Input: part model. Units: mm. Frame: model coordinates. Coordinates: 2 decimals unless noted, no trailing zeros. Write each loop counter-clockwise with the first axis right and the second up, starting at its lowest first coordinate (ties: lowest second). Pieces come first, ordered by that corner, then holes. Notation, with made-up numbers: (68, 12) - (115, 12) arc R24 ccw to (115, 35) - close; hole circle Ø10 at (38, -28). An arc over 180 degrees is marked (long way). Use CSV: the item, a comma, the result in double quotes.
Autodesk Inventor part; units mm, degrees
ref_plane "YZ Plane" through (0, 0, 0) normal (1, 0, 0) x (0, 1, 0)
ref_plane "XZ Plane" through (0, 0, 0) normal (0, 1, 0) x (-1, 0, 0)
ref_plane "XY Plane" through (0, 0, 0) normal (0, 0, 1) x (1, 0, 0)
sketch "Sketch1" plane through (0, 0, 0) normal (0, 1, 0) x (-1, 0, 0)
  line L0 (0, 0) -> (152.4, 0)
  line L1 (152.4, 0) -> (152.4, 203.2)
  line L2 (152.4, 203.2) -> (0, 203.2)
  line L3 (0, 203.2) -> (0, 0)
  circle A0 centre (12.7, 190.5) radius 7.9375
  circle A1 centre (139.7, 190.5) radius 7.9375
  circle A2 centre (139.7, 12.7) radius 7.9375
  circle A3 centre (12.7, 12.7) radius 7.9375
  circle A4 centre (114.3, 190.5) radius 3.302
  circle A5 centre (38.1, 190.5) radius 3.302
  circle A6 centre (114.3, 12.7) radius 3.302
  circle A7 centre (38.1, 12.7) radius 3.302
  circle A8 centre (139.7, 139.7) radius 3.302
  circle A9 centre (139.7, 63.5) radius 3.302
  circle A10 centre (20.32, 168.148) radius 1.524
  circle A11 centre (20.32, 153.924) radius 1.524
  circle A12 centre (20.32, 128.524) radius 1.524
  circle A13 centre (20.32, 114.3) radius 1.524
  circle A14 centre (20.32, 88.9) radius 1.524
  circle A15 centre (20.32, 74.676) radius 1.524
  circle A16 centre (20.32, 49.276) radius 1.524
  circle A17 centre (20.32, 35.052) radius 1.524
  line L4 (152.4, 203.2) -> (139.7, 203.2)
  line L5 (139.7, 203.2) -> (139.7, 200.025)
  line L6 (139.7, 200.025) -> (152.4, 200.025)
  line L7 (152.4, 200.025) -> (152.4, 203.2)
  line L8 (127, 203.2) -> (114.3, 203.2)
  line L9 (114.3, 203.2) -> (114.3, 200.025)
  line L10 (114.3, 200.025) -> (127, 200.025)
  line L11 (127, 200.025) -> (127, 203.2)
  line L12 (101.6, 203.2) -> (88.9, 203.2)
  line L13 (88.9, 203.2) -> (88.9, 200.025)
  line L14 (88.9, 200.025) -> (101.6, 200.025)
  line L15 (101.6, 200.025) -> (101.6, 203.2)
  line L16 (76.2, 203.2) -> (63.5, 203.2)
  line L17 (63.5, 203.2) -> (63.5, 200.025)
  line L18 (63.5, 200.025) -> (76.2, 200.025)
  line L19 (76.2, 200.025) -> (76.2, 203.2)
  line L20 (50.8, 203.2) -> (38.1, 203.2)
  line L21 (38.1, 203.2) -> (38.1, 200.025)
  line L22 (38.1, 200.025) -> (50.8, 200.025)
  line L23 (50.8, 200.025) -> (50.8, 203.2)
  line L24 (25.4, 203.2) -> (12.7, 203.2)
  line L25 (12.7, 203.2) -> (12.7, 200.025)
  line L26 (12.7, 200.025) -> (25.4, 200.025)
  line L27 (25.4, 200.025) -> (25.4, 203.2)
  line L28 (152.4, 0) -> (139.7, 0)
  line L29 (139.7, 0) -> (139.7, 3.175)
  line L30 (139.7, 3.175) -> (152.4, 3.175)
  line L31 (152.4, 3.175) -> (152.4, 0)
  line L32 (127, 0) -> (114.3, 0)
  line L33 (114.3, 0) -> (114.3, 3.175)
  line L34 (114.3, 3.175) -> (127, 3.175)
  line L35 (127, 3.175) -> (127, 0)
  line L36 (101.6, 0) -> (88.9, 0)
  line L37 (88.9, 0) -> (88.9, 3.175)
  line L38 (88.9, 3.175) -> (101.6, 3.175)
  line L39 (101.6, 3.175) -> (101.6, 0)
  line L40 (76.2, 0) -> (63.5, 0)
  line L41 (63.5, 0) -> (63.5, 3.175)
  line L42 (63.5, 3.175) -> (76.2, 3.175)
  line L43 (76.2, 3.175) -> (76.2, 0)
  line L44 (50.8, 0) -> (38.1, 0)
  line L45 (38.1, 0) -> (38.1, 3.175)
  line L46 (38.1, 3.175) -> (50.8, 3.175)
  line L47 (50.8, 3.175) -> (50.8, 0)
  line L48 (25.4, 0) -> (12.7, 0)
  line L49 (12.7, 0) -> (12.7, 3.175)
  line L50 (12.7, 3.175) -> (25.4, 3.175)
  line L51 (25.4, 3.175) -> (25.4, 0)
  line L52 (152.4, 187.325) -> (149.225, 187.325)
  line L53 (149.225, 187.325) -> (149.225, 174.625)
  line L54 (149.225, 174.625) -> (152.4, 174.625)
  line L55 (152.4, 174.625) -> (152.4, 187.325)
  line L56 (152.4, 161.925) -> (149.225, 161.925)
  line L57 (149.225, 161.925) -> (149.225, 149.225)
  line L58 (149.225, 149.225) -> (152.4, 149.225)
  line L59 (152.4, 149.225) -> (152.4, 161.925)
  line L60 (152.4, 136.525) -> (149.225, 136.525)
  line L61 (149.225, 136.525) -> (149.225, 123.825)
  line L62 (149.225, 123.825) -> (152.4, 123.825)
  line L63 (152.4, 123.825) -> (152.4, 136.525)
  line L64 (152.4, 107.95) -> (149.225, 107.95)
  line L65 (149.225, 107.95) -> (149.225, 95.25)
  line L66 (149.225, 95.25) -> (152.4, 95.25)
  line L67 (152.4, 95.25) -> (152.4, 107.95)
  line L68 (152.4, 79.375) -> (149.225, 79.375)
  line L69 (149.225, 79.375) -> (149.225, 66.675)
  line L70 (149.225, 66.675) -> (152.4, 66.675)
  line L71 (152.4, 66.675) -> (152.4, 79.375)
  line L72 (152.4, 53.975) -> (149.225, 53.975)
  line L73 (149.225, 53.975) -> (149.225, 41.275)
  line L74 (149.225, 41.275) -> (152.4, 41.275)
  line L75 (152.4, 41.275) -> (152.4, 53.975)
  line L76 (152.4, 28.575) -> (149.225, 28.575)
  line L77 (149.225, 28.575) -> (149.225, 15.875)
  line L78 (149.225, 15.875) -> (152.4, 15.875)
  line L79 (152.4, 15.875) -> (152.4, 28.575)
  line L80 (0, 147.574) -> (0, 134.874)
  line L81 (0, 134.874) -> (3.175, 134.874)
  line L82 (3.175, 134.874) -> (3.175, 147.574)
  line L83 (3.175, 147.574) -> (0, 147.574)
  line L84 (0, 107.95) -> (0, 95.25)
  line L85 (0, 95.25) -> (3.175, 95.25)
  line L86 (3.175, 95.25) -> (3.175, 107.95)
  line L87 (3.175, 107.95) -> (0, 107.95)
  line L88 (0, 55.626) -> (0, 68.326)
  line L89 (0, 68.326) -> (3.175, 68.326)
  line L90 (3.175, 68.326) -> (3.175, 55.626)
  line L91 (3.175, 55.626) -> (0, 55.626)
  dimension "d0" = 152.4
  dimension "d1" = 203.2
  dimension "d40" = 15.875
  dimension "d41" = 15.875
  dimension "d42" = 15.875
  dimension "d43" = 15.875
  dimension "d44" = 12.7
  dimension "d45" = 12.7
  dimension "d46" = 12.7
  dimension "d47" = 12.7
  dimension "d48" = 12.7
  dimension "d49" = 12.7
  dimension "d50" = 12.7
  dimension "d51" = 12.7
  dimension "d52" = 177.8
  dimension "d53" = 127
  dimension "d54" = 6.604
  dimension "d55" = 6.604
  dimension "d56" = 25.4
  dimension "d57" = 25.4
  dimension "d58" = 12.7
  dimension "d59" = 12.7
  dimension "d60" = 6.604
  dimension "d61" = 6.604
  dimension "d62" = 12.7
  dimension "d63" = 12.7
  dimension "d64" = 25.4
  dimension "d65" = 25.4
  dimension "d66" = 6.604
  dimension "d67" = 6.604
  dimension "d68" = 50.8
  dimension "d69" = 50.8
  dimension "d70" = 12.7
  dimension "d71" = 12.7
  dimension "d72" = 3.048
  dimension "d73" = 3.048
  dimension "d74" = 3.048
  dimension "d75" = 3.048
  dimension "d76" = 3.048
  dimension "d77" = 3.048
  dimension "d78" = 20.32
  dimension "d79" = 20.32
  dimension "d80" = 20.32
  dimension "d81" = 20.32
  dimension "d82" = 20.32
  dimension "d83" = 20.32
  dimension "d84" = 22.352
  dimension "d85" = 14.224
  dimension "d86" = 25.4
  dimension "d87" = 14.224
  dimension "d88" = 25.4
  dimension "d89" = 14.224
  dimension "d90" = 3.048
  dimension "d91" = 3.048
  dimension "d92" = 25.4
  dimension "d93" = 14.224
  dimension "d97" = 12.7
  dimension "d98" = 3.175
  dimension "d99" = 12.7
  dimension "d100" = 3.175
  dimension "d101" = 12.7
  dimension "d102" = 3.175
  dimension "d103" = 12.7
  dimension "d104" = 3.175
extrude "Extrusion4" add sketch "Sketch1" along normal blind 25.4 contours L3 L91 L90 L89 L85 L86 L87 L81 L82 L83 L2 L25 L26 L27 L21 L22 L23 L17 L18 L19 L13 L14 L15 L9 L10 L11 L5 L6 L1 L52 L53 L54 L56 L57 L58 L60 L61 L62 L64 L65 L66 L68 L69 L70 L72 L73 L74 L76 L77 L78 L30 L29 L0 L35 L34 L33 L39 L38 L37 L43 L42 L41 L47 L46 L45 L51 L50 L49
properties part number "CasingBottomWithSlotsInFront"
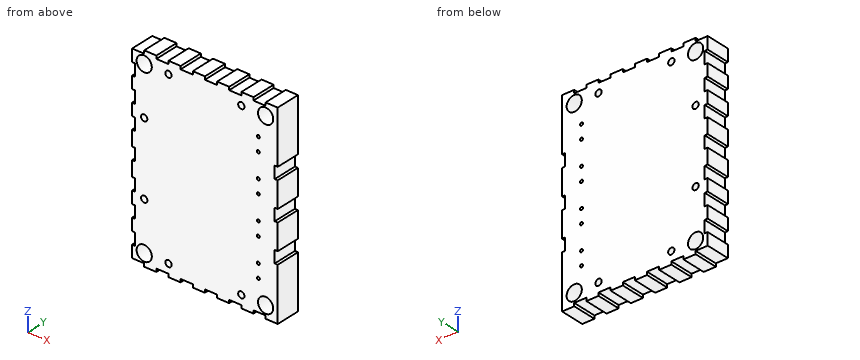
(1) Cut plane A-A on z = 63.5. Return loops of the section in (x, y) (3 decimals), and give its area (3 significant figures).
Check values:
outline,"(-152.4, 0) - (-143.002, 0) - (-143.002, 25.4) - (-152.4, 25.4) - close; (-136.398, 0) - (-3.175, 0) - (-3.175, 25.4) - (-136.398, 25.4) - close"
area,"3,620 mm^2"
(2) Cut plane B-B on z = 190.5. Return loops of the section in (x, y).
Check values:
outline,"(-152.4, 0) - (-147.64, 0) - (-147.64, 25.4) - (-152.4, 25.4) - close; (-131.76, 0) - (-117.6, 0) - (-117.6, 25.4) - (-131.76, 25.4) - close; (-111, 0) - (-41.4, 0) - (-41.4, 25.4) - (-111, 25.4) - close; (-34.8, 0) - (-20.64, 0) - (-20.64, 25.4) - (-34.8, 25.4) - close; (-4.76, 0) - (0, 0) - (0, 25.4) - (-4.76, 25.4) - close"
(3) Pin query (flat end, axial travel): pin 1 Ø6.5 at (y, z) = (17, 101) entering from -X (3 decimals); pin 2 Ø1.6 at (x, y) = (-150.5, 11.5) entering from +Z (3 decimals); pin 3 Ø2.5 at (x, y) = (-150, 16) entering from -Z (3 decimals). Return the tip coordinate at first contact, or that it passes through.
Check values:
pin 1,"x = -149.225"
pin 2,"z = 200.025"
pin 3,"z = 3.175"
(4) Cut plane C-C on y = 9.25. State how many separate pieces and enclosed holes the cut face has, and give its area (3 significant figures).
Check values:
separate pieces,"1"
enclosed holes,"18"
area,"29,000 mm^2"
(5) Ray query, probe 1 along Z at (x, y) = (-36.5, 22.25); probe 2 along X at (y, z) = (8.25, 139.7) (3 decimals); probe 3 along Z at (x, y) = (-14, 3) (3 decimals). Return the intervals inside material, ascending. Write a range as from..to.
Check values:
probe 1,"0..9.81, 15.59..187.61, 193.39..203.2"
probe 2,"-152.4..-143.002, -136.398..-3.175"
probe 3,"3.175..4.87, 20.53..182.67, 198.33..200.025"
